Read the model definition and answer for the solid it produces. Units are mm, in the model's axes. Give positions to 0.01 mm unless a question says otherwise; leave off trailing zeros. Loops run counter-clockwise (first coordinate to the right, second up) from the corner with the lowest first, then second, coordinate; pieces in that order, holes last. Notation, with made-up numbers: (25.5, 17) - (71.5, 17) arc R18 ccw to (71.5, 28) - close; hole circle Ø1 at (20, -36). An arc over 180 degrees is marked (long way). Write each question's results on one line, items separated by ' | '. Start each with the question number.
Q1. The part is cut by section B-B, the plane z = 22. Write down the section's boundary in (x, y).
Q2. Given pin 1 (4 mm diameter, centred on x = 6, z = 19, fed in from +Y); pin 2 (16.5 mm diameter, centred on x = -4, z = 4.5, fed in from -Y); pin 3 (3 mm diameter, centred on x = -6, y = 9, fed in from +Z); pin 4 (10.5 mm diameter, centred on x = 0, z = 0, fed in from +Y) (3 decimals), each flat-ended and moving along its own axis, determine where each tip first touches the part or whether it passes through.
Q3. Find the intervals of material crossed by line 1 (Z direction, x = 0, y = 0) (3 decimals); line 2 (Z direction, x = 0, y = 1.25) (3 decimals); line 3 (Z direction, x = 6.5, y = -7), in increasing order. Write a range as from..to.
Q4. The part is cut by section A-A, the plane z = 0. Write down the section's boundary in (x, y) (3 decimals).
Q5. Determine the mould class of faces 1 (the flat face through (1, -3, -10)), 2 (the cylindrical face through (-0.415, -0.042, -10.367)), 3 (the flat face through (1, 0, 34.961)) for opening direction Z: +Z half, -Z half, draft (parallel to the pull), parting line (faces both ways), or undercut.
```python
from build123d import *

# Parameters (mm, degrees)
F0_R          = 8.875
F3_DEPTH      = 3
F3_DEPTH_BACK = 3
F4_SIZE       = 1
F5_R          = 0.5
F6_DEPTH      = 0.43
F7_DEPTH      = 0.82


with BuildPart() as f2:
    # F0 (on Front) → F2 (revolve)
    with BuildSketch(Plane.XZ):
        with BuildLine():
            ThreePointArc((0, 10.375), (1.4661242569, 10.2708862647), (2.9028232275, 9.9606346339))
            ThreePointArc((2.9028232275, 9.9606346339), (9.4069705736, 10.9259285589), (15, 14.3833476682))
            Line((15, 14.3833476682), (3.7, 34.9606346339))
            Line((3.7, 34.9606346339), (0, 34.9606346339))
            Line((0, 34.9606346339), (0, 10.375))
        make_face()
    revolve(axis=Axis((0, 0, 0), (0, 0, 1)))

    # F0 (on Front) → F3 (join, two sides)
    with BuildSketch(Plane.XZ) as f3_sk:
        with BuildLine():
            ThreePointArc((0, 10.375), (-7.3362328548, -7.3362328548), (10.375, 0))
            ThreePointArc((10.375, 0), (8.2993197307, 6.2259069225), (2.9028232275, 9.9606346339))
            Line((2.9028232275, 9.9606346339), (0, 9.9606346339))
            Line((0, 9.9606346339), (0, 10.375))
        make_face()
        Circle(F0_R, mode=Mode.SUBTRACT)
        with BuildLine():
            Line((0, 9.9606346339), (2.9028232275, 9.9606346339))
            ThreePointArc((2.9028232275, 9.9606346339), (1.4661242569, 10.2708862647), (0, 10.375))
            Line((0, 10.375), (0, 9.9606346339))
        make_face()
    extrude(amount=F3_DEPTH)
    extrude(f3_sk.sketch, amount=-F3_DEPTH_BACK)

    # F4
    f4_edges = [f2.edges().sort_by_distance(p)[0] for p in [
        (-8.875, -3, 0),
        (-8.875, 3, 0),
    ]]
    chamfer(f4_edges, length=F4_SIZE)

    # F5 (on face) → F6 (cut)
    with BuildSketch(Plane.XY.offset(34.9606346339)):
        with BuildLine():
            ThreePointArc((0.0041443855, 1.7524251654), (-0.4908303614, 1.5473999123), (-0.6958556145, 1.0524251654))
            Line((-0.6958556145, 1.0524251654), (-0.6958556145, -1.0399995122))
            ThreePointArc((-0.6958556145, -1.0399995122), (-0.4908303614, -1.534974259), (0.0041443855, -1.7399995122))
            ThreePointArc((0.0041443855, -1.7399995122), (0.4991191323, -1.534974259), (0.7041443855, -1.0399995122))
            Line((0.7041443855, -1.0399995122), (0.7041443855, 1.0524251654))
            ThreePointArc((0.7041443855, 1.0524251654), (0.4991191323, 1.5473999123), (0.0041443855, 1.7524251654))
        make_face()
        with Locations((0.0021327037, 0.0014704808)):
            Circle(F5_R, mode=Mode.SUBTRACT)
        with BuildLine():
            ThreePointArc((-2.2493049037, 1.7524251654), (-2.7442796505, 1.5473999123), (-2.9493049037, 1.0524251654))
            Line((-2.9493049037, 1.0524251654), (-2.9493049037, -1.0399995122))
            ThreePointArc((-2.9493049037, -1.0399995122), (-2.7442796505, -1.534974259), (-2.2493049037, -1.7399995122))
            ThreePointArc((-2.2493049037, -1.7399995122), (-1.7543301568, -1.534974259), (-1.5493049037, -1.0399995122))
            Line((-1.5493049037, -1.0399995122), (-1.5493049037, 1.0524251654))
            ThreePointArc((-1.5493049037, 1.0524251654), (-1.7543301568, 1.5473999123), (-2.2493049037, 1.7524251654))
        make_face()
        with BuildLine():
            ThreePointArc((2.2571443855, 1.7524251654), (1.7621696386, 1.5473999123), (1.5571443855, 1.0524251654))
            Line((1.5571443855, 1.0524251654), (1.5571443855, -1.0399995122))
            ThreePointArc((1.5571443855, -1.0399995122), (1.7621696386, -1.534974259), (2.2571443855, -1.7399995122))
            ThreePointArc((2.2571443855, -1.7399995122), (2.7521191323, -1.534974259), (2.9571443855, -1.0399995122))
            Line((2.9571443855, -1.0399995122), (2.9571443855, 1.0524251654))
            ThreePointArc((2.9571443855, 1.0524251654), (2.7521191323, 1.5473999123), (2.2571443855, 1.7524251654))
        make_face()
    extrude(amount=-F6_DEPTH, mode=Mode.SUBTRACT)

    # F7 (cut): a face of the model
    f7_faces = [f2.faces().sort_by_distance(p)[0] for p in [
        (0.0021327037, 0.0014704808, 34.9606346339),
    ]]
    extrude(f7_faces, amount=-F7_DEPTH, mode=Mode.SUBTRACT)


solid = f2.part
```
Check sheet entries:
1) outline: circle Ø21.63 at (0, 0)
2) pin 1: stops at y = 12.45 | pin 2: stops at y = -12.53 | pin 3: stops at z = 24.73 | pin 4: passes through
3) line 1: z = -10.375..-8.875, 8.875..34.141 | line 2: z = -10.375..-8.875, 8.875..34.531 | line 3: z = 10.98..24.3
4) outline: (-10.375, -3) - (-9.875, -3) - (-8.875, -2) - (-8.875, 2) - (-9.875, 3) - (-10.375, 3) - close; (8.875, -2) - (9.875, -3) - (10.375, -3) - (10.375, 3) - (9.875, 3) - (8.875, 2) - close
5) face 1: draft | face 2: undercut | face 3: +Z half
